Autodesk Inventor part; units mm, degrees
ref_plane "Plano inicial" through (0, 0, 0) normal (0, 0, 1) x (1, 0, 0)
ref_plane "Plano final" through (0, 0, 120) normal (0, 0, 1) x (1, 0, 0)
ref_plane "Plano de trabalho4" through (-15, 0, 0) normal (0.7071, 0, -0.7071) x (-0.7071, 0, -0.7071)
ref_plane "Plano inicial" through (0, 0, 0) normal (0, 0, 1) x (1, 0, 0)
ref_plane "Plano final" through (0, 0, 120) normal (0, 0, 1) x (1, 0, 0)
sketch "Esboço" plane through (0, 0, 0) normal (0, 0, 1) x (1, 0, 0)
  line L0 (-15, -11) -> (-15, 11)
  line L1 (-11, 15) -> (11, 15)
  line L2 (15, 11) -> (15, -11)
  line L3 (11, -15) -> (-11, -15)
  arc A0 (-15, -11) -> (-11, -15) centre (-11, -11) ccw
  arc A1 (15, 11) -> (11, 15) centre (11, 11) ccw
  arc A2 (-11, 15) -> (-15, 11) centre (-11, 11) ccw
  arc A3 (11, -15) -> (15, -11) centre (11, -11) ccw
  arc A4 (-11, 13) -> (-13, 11) centre (-11, 11) ccw
  line L4 (-11, 13) -> (11, 13)
  arc A5 (13, 11) -> (11, 13) centre (11, 11) ccw
  line L5 (13, 11) -> (13, -11)
  arc A6 (11, -13) -> (13, -11) centre (11, -11) ccw
  line L6 (11, -13) -> (-11, -13)
  arc A7 (-13, -11) -> (-11, -13) centre (-11, -11) ccw
  line L7 (-13, -11) -> (-13, 11)
  line L8 (0, 22.1598) -> (0, -22.1598) construction
  line L9 (-22.1598, 0) -> (22.1598, 0) construction
  dimension "d7" = 4
  dimension "d9" = 30
  dimension "d11" = 30
  dimension "d12" = 2
  dimension "d15" = 15
  dimension "d16" = 15
extrude "Corpo" add sketch "Esboço" along normal up to surface (120 mm away) from surface at 0
sketch "Sketch3" plane through (0, 0, 0) normal (0, 0, 1) x (1, 0, 0)
  line L0 (0, 0) -> (10, 0)
ref_plane "Work Plane3" through (0, 0, 0) normal (0, -1, 0) x (1, 0, 0)
sketch "Sketch4" plane through (0, 0, 0) normal (0, -1, 0) x (1, 0, 0)
  line L0 (-2, 0) -> (12, 0)
  line L1 (-2, 120) -> (12, 120)
  dimension "d18" = 120
ref_plane "Plano de trabalho4" through (-15, 0, 0) normal (0.7071, 0, -0.7071) x (-0.7071, 0, -0.7071)
split "Dividir1" plane through (-15, 0, 0) removes the side toward (0.7071, 0, -0.7071)
ref_plane "Plano de trabalho5" through (-15, 0, 120) normal (0.7071, 0, 0.7071) x (0.7071, 0, -0.7071)
split "Dividir2" plane through (-15, 0, 120) removes the side toward (0.7071, 0, 0.7071)
equation "\"d7\" = G_IR"
equation "\"d9\" = G_W"
equation "\"d11\" = G_H"
equation "\"d12\" = G_T"
equation "\"d15\" = 0.5 * d9"
equation "\"d16\" = 0.5 * d11"
equation "\"d3\" = G_L"
equation "\"G_W\" = 30"
equation "\"G_H\" = 30"
equation "\"G_T\" = 2"
equation "\"G_IR\" = 4"
equation "\"G_L\" = d18"
equation "\"G_OFFSET_START\" = 0"
equation "\"G_OFFSET_END\" = 0"
properties part number "ISO 10799-2 - 30x30x2 - 120" material "Aço, suave"
Part model, mm, in its own coordinate system. A direction names the side the tool comes from. Give positions to 0.01 mm unless a question says otherwise; leave off trailing zeros. Order: outer loops, then holes, each group sorted by start corner. A loop starts at its lowest first (then second) coordinate and runs counter-clockwise, first axis right, second up. Notation, with made-up numbers: M 26,12.5 L 34,12.5 A19 cw 34,16.5 Z; hole C 81,-2 d11. An arc over 180 degrees is marked long. Use a Markdown table: item, result. Add a question column.
(1) 3-axis set-ups, long thin cutter, end or side, ignore diameter. For faces 1 (the face through (13, 0, 60)), 2 (the face through (0, -14, 105)): which of +Z, -Z, +X, -X, +Y, -Y reach the whole face in a straight line?
(2) Probe line 1 along Y through (x, z) = (-7, 48); line 2 along X through (y, z) = (-4, 104). List the from-to ranges inside material, lowest first. Write a range as [from, to].
(3) Saw through at B-B, the plane y = 1.75. Give the cut face in (x, z).
(4) Saw through at C-C, the plane z = 39.5. Give the cut face in (x, y), and give its area (3 significant figures).
(5) Mould opens along X. For faces 3 (the face through (-13.859, 13.797, 59.16)), 4 (the face through (13.859, -13.797, 59.524)), 5 (the face through (12.43, -12.4, 59.52)) say: +X half, -X half, draft (parallel to the pull), parting line (faces both ways), or undercut.
(6) Saw through at A-A, the plane x = 9.25. Give the cut face in (y, z).
(7) Saw through at D-D, the plane z = 101. Give the cut face in (x, y).
(8) Drop flat-ended pins along their axis: P1, Ø8, axis at x = 9.5, y = 9.5, coming from the +Z side; P2, Ø12, axis at x = 1.5, y = -11.5, coming from the +Z side; P3, Ø3, axis at x = -10, y = -4, coming from the +Z side. Give the stop position or say it passes through.
Answer key:
| question | item | result |
|---|---|---|
| 1 | face 1 | +Z, -Z |
| 1 | face 2 | +Z, +X, +Y, -Y |
| 2 | line 1 | [-15, -13], [13, 15] |
| 2 | line 2 | [-15, -13] |
| 3 | outline | M -15,0 L -13,2 L -13,118 L -15,120 Z; M 13,28 L 15,30 L 15,90 L 13,92 Z |
| 4 | outline | M -15,-11 A4 ccw -11,-15 L 11,-15 A4 ccw 15,-11 L 15,11 A4 ccw 11,15 L -11,15 A4 ccw -15,11 Z; hole M -13,-11 A2 ccw -11,-13 L 11,-13 A2 ccw 13,-11 L 13,11 A2 ccw 11,13 L -11,13 A2 ccw -13,11 Z |
| 4 | area | 214 mm^2 |
| 5 | face 3 | -X half |
| 5 | face 4 | +X half |
| 5 | face 5 | undercut |
| 6 | outline | M -15,24.25 L -13,24.25 L -13,95.75 L -15,95.75 Z; M 13,24.25 L 15,24.25 L 15,95.75 L 13,95.75 Z |
| 7 | outline | M -15,-11 A4 ccw -11,-15 L 4,-15 L 4,-13 L -11,-13 A2 cw -13,-11 L -13,11 A2 cw -11,13 L 4,13 L 4,15 L -11,15 A4 ccw -15,11 Z |
| 8 | P1 | z = 97.44 |
| 8 | P2 | z = 109.31 |
| 8 | P3 | through |
